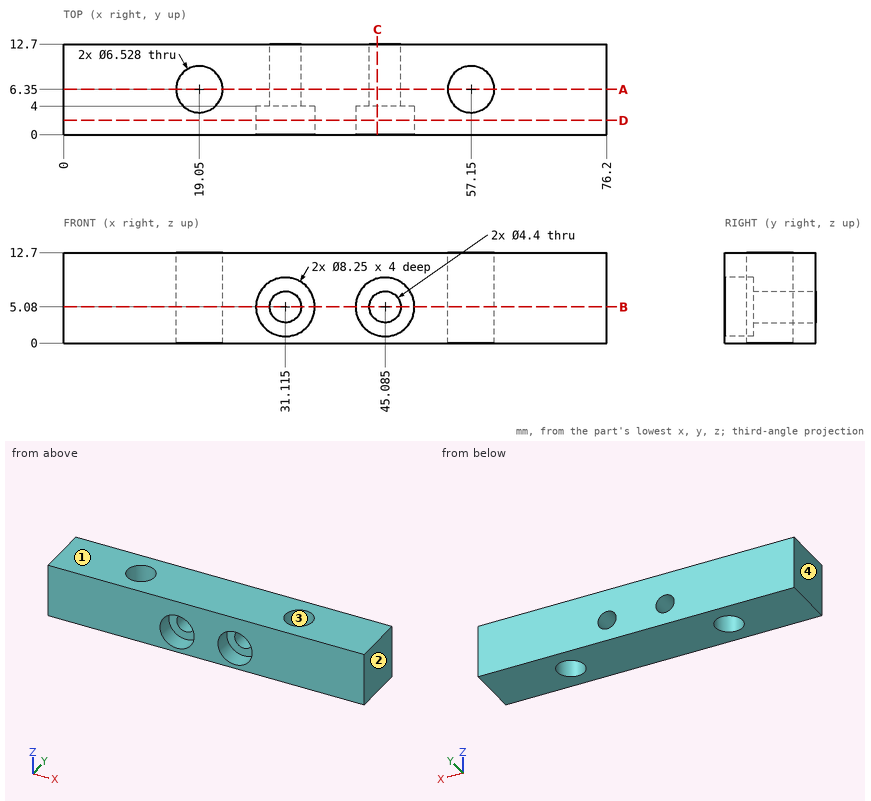
Check sheet for the drawn part. Datum: minimum x, y, z corner. Units: mm. Round coordinates to 2 decimals unless told otherwise and drop trailing zeros. Loops run counter-clockwise (first coordinate to the right, second up) from the corner with the lowest first, then second, coordinate; pieces in that order, holes last. Notation, with made-up numbers: M 61.25,2 L 111.25,2 A17 cw 111.25,27 Z; hole C 57.5,61.25 d2. An arc over 180 degrees is marked long. One line per question, with ' | ' between items. Start each with the question number.
Item 1: Release check for a two-part mould opening along X. For the marked faces 1, 2, 3 and 4 record: released by +X, released by -X, zero draft, split by the parting line, or undercut.
Item 2: Section check A-A (y = 6.35). Record the boundary of the cut face in (x, z) (1 decimal).
Item 3: Section check D-D (y = 2). Record the boundary of the cut face in (x, z) (3 decimals).
Item 4: Section check B-B (z = 5.08). State how many separate pieces and enclosed holes the cut face has, and give its area (3 significant figures).
Item 5: Gauge pin test, flat ends, axial feed: pin 1 Ø4 at (x, z) = (59, 6) entering from -Y; pin 2 Ø6.5 at (x, z) = (44.5, 5) entering from -Y. Record the tip position at first contact, or that the pin passes through.
Item 6: Section check C-C (x = 44). Record the boundary of the cut face in (y, z).
Item 7: Scan lines: probe 1 along Y at (x, z) = (19, 5.75); probe 2 along X at (y, z) = (6, 1.25) (1 decimal); probe 3 along X at (y, z) = (8.25, 8.5). Record each from-to range of solid material in increasing order.
Worked out:
1) face 1: zero draft | face 2: released by +X | face 3: undercut | face 4: released by -X
2) outline: M 0,0 L 15.8,0 L 15.8,12.7 L 0,12.7 Z; M 22.3,0 L 53.9,0 L 53.9,12.7 L 22.3,12.7 Z; M 60.4,0 L 76.2,0 L 76.2,12.7 L 60.4,12.7 Z; hole C 31.1,5.1 d4.4; hole C 45.1,5.1 d4.4
3) outline: M 0,0 L 76.2,0 L 76.2,12.7 L 0,12.7 Z; hole C 31.115,5.08 d8.25; hole C 45.085,5.08 d8.25
4) separate pieces: 3 | enclosed holes: 2 | area: 758 mm^2
5) pin 1: y = 0 | pin 2: y = 4
6) outline: M 0,0 L 12.7,0 L 12.7,3.17 L 4,3.17 L 4,1.1 L 0,1.1 Z; M 0,9.06 L 4,9.06 L 4,6.99 L 12.7,6.99 L 12.7,12.7 L 0,12.7 Z
7) probe 1: 0 to 3.09, 9.61 to 12.7 | probe 2: 0 to 15.8, 22.3 to 53.9, 60.4 to 76.2 | probe 3: 0 to 16.4, 21.7 to 54.5, 59.8 to 76.2
